Can you work these out from the drawing? Everything is in mm from the part's minimum corner. A direction names the side the tool comes from. Give positions to 0.01 mm unless a question says otherwise; leave off trailing zeros. Order: outer loops, then holes, each group sorted by start corner. A loop starts at its lowest first (then second) coordinate and runs counter-clockwise, first axis right, second up. Notation, with made-up numbers: (-8, 48) -> (-3, 48) arc R8 cw to (-3, 52) -> close; hole circle Ø1 at (39, 75.5). An arc over 180 degrees is marked (long way). Answer as CSV lines item,"result". Start each with the question number.
(1) I want a section at D-D (y = 13). Please give me the cut outline in (x, z) (1 decimal), plus the area to 3 significant figures.
(2) I want a section at C-C (x = 24.5). Please give me the cut outline in (y, z) (1 decimal).
(3) I want a section at A-A (z = 14.5). Please give me the cut outline in (x, y).
(4) Will these pins go through, and if not, where does the flat tip stop? pin 1 Ø1.1 at (y, z) = (1, 45) entering from -X; pin 2 Ø20.5 at (x, y) = (44.5, 50.5) entering from +Z; pin 3 Ø1.1 at (x, y) = (17.5, 74.5) entering from +Z.
(5) On a 3-axis mill with a long thin cutter (end or side, diameter ignored), from which of +Z, -Z, +X, -X, +Y, -Y can I reach the whole of each face in a straight line? I mean the marked faces 1 and 2. Say none if no direction works.
(6) We'd pull the mould along Y, two halves only. Please class the marked faces 3, 4 and 5: released by +Y, released by -Y, zero draft, split by the parting line, or undercut.
(7) I want a section at B-B (z = 40.5). Please give me the cut outline in (x, y).
(8) I need wall thicknesses on L1, parallel to Y at x = 29.5, z = 12; L2, parallel to X at y = 73, z = 22; L3, parallel to Z at x = 32, y = 51.5 (1 decimal). Which ranges of each line are inside material? Lowest first, please.
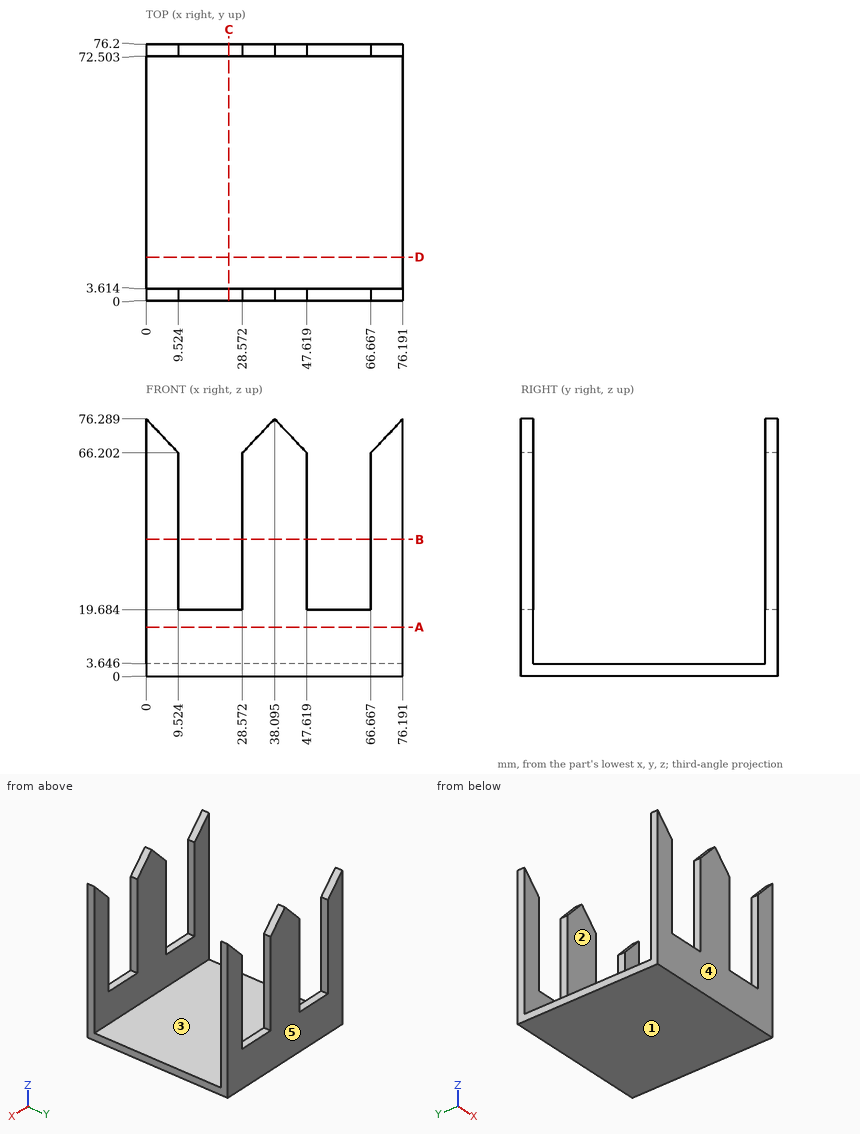
Final values:
1,outline,"(0, 0) -> (76.2, 0) -> (76.2, 3.6) -> (0, 3.6) -> close"
1,area,"278 mm²"
2,outline,"(0, 0) -> (76.2, 0) -> (76.2, 19.7) -> (72.5, 19.7) -> (72.5, 3.6) -> (3.6, 3.6) -> (3.6, 19.7) -> (0, 19.7) -> close"
3,outline,"(0, 0) -> (76.19, 0) -> (76.19, 3.61) -> (0, 3.61) -> close; (0, 72.5) -> (76.19, 72.5) -> (76.19, 76.2) -> (0, 76.2) -> close"
4,pin 1,"x = 0"
4,pin 2,"z = 3.65"
4,pin 3,"z = 19.68"
5,face 1,"-Z, +X, -X, +Y, -Y"
5,face 2,"+Z, +X, -X"
6,face 3,"undercut"
6,face 4,"released by -Y"
6,face 5,"released by +Y"
7,outline,"(0, 0) -> (9.52, 0) -> (9.52, 3.61) -> (0, 3.61) -> close; (0, 72.5) -> (9.52, 72.5) -> (9.52, 76.2) -> (0, 76.2) -> close; (28.57, 0) -> (47.62, 0) -> (47.62, 3.61) -> (28.57, 3.61) -> close; (28.57, 72.5) -> (47.62, 72.5) -> (47.62, 76.2) -> (28.57, 76.2) -> close; (66.67, 0) -> (76.19, 0) -> (76.19, 3.61) -> (66.67, 3.61) -> close; (66.67, 72.5) -> (76.19, 72.5) -> (76.19, 76.2) -> (66.67, 76.2) -> close"
8,L1,"0 to 3.61, 72.5 to 76.2"
8,L2,"0 to 9.52, 28.57 to 47.62, 66.67 to 76.19"
8,L3,"0 to 3.6"
